Check sheet for the drawn part. Datum: minimum x, y, z corner. Units: mm. A direction names the side the tool comes from. Round coordinates to 2 decimals unless told otherwise and drop trailing zeros. Write each loop counter-clockwise with the first axis right and the second up, starting at its lowest first coordinate (ties: lowest second). Pieces come first, ordered by that corner, then holes. Notation, with made-up numbers: (-1.75, 18.25) - (42.25, 18.25) arc R28 ccw to (42.25, 42.25) - close; hole circle Ø4 at (-20.5, -22). An arc over 180 degrees is marked (long way). Answer as a JSON object with one key per item and string values. Group by question number.
Item 1: Sectioned sample at D-D on x = 12. Record the boundary of the cut face in (y, z) (1 decimal).
Item 2: Release check for a two-part mould opening along X. For the marked faces 1, 2 and 3 record: pulls with the +X half, pulls with the -X half, needs draft (parallel to the pull), parting line crosses it, or undercut.
Item 3: Sectioned sample at B-B on y = 4.75. Record the boundary of the cut face in (x, z).
Item 4: Set-up check for the marked faces 4, 5 and 6: record each of +Z, -Z, +X, -X, +Y, -Y from which the full face is reachable in a straight line by a thin tool's end or side.
Item 5: Sectioned sample at A-A on z = 5. Record the boundary of the cut face in (x, y).
Item 6: Thickness scan on line 1 (Y direction, x = 10, z = 12); line 2 (X direction, y = 9.5, z = 14) (1 decimal); line 3 (Z direction, x = 31, y = 17.75). Record the ranges inside material, lowest first.
Item 7: Gauge pin test, flat ends, axial feed: P1, Ø1.5, axis at y = 13, z = 6.5, coming from the -X side; P2, Ø11, axis at x = 29, y = 17.5, coming from the -Z side; P3, Ø1.5, axis at x = 38.5, z = 16, coming from the -Y side; P4, Ø0.6, axis at x = 21.5, z = 33.5, coming from the -Y side. Record the tip position at first contact, or that the pin passes through.
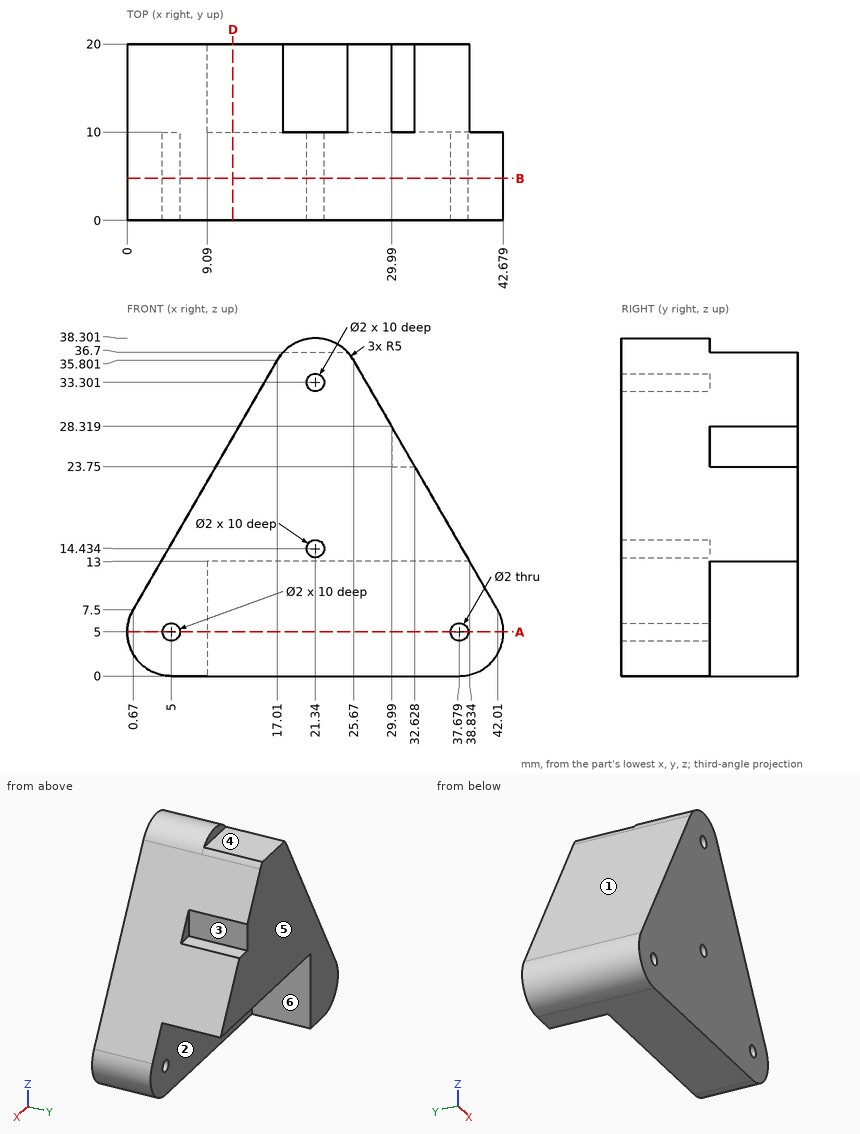
Completed:
{
 "1": {"outline": "(0, 0) - (10, 0) - (10, 13) - (20, 13) - (20, 27.1) - (0, 27.1) - close"},
 "2": {"face 1": "pulls with the -X half", "face 2": "needs draft", "face 3": "pulls with the +X half"},
 "3": {"outline": "(0.67, 7.5) arc R5 ccw to (5, 0) - (37.68, 0) arc R5 ccw to (42.01, 7.5) - (25.67, 35.8) arc R5 ccw to (17.01, 35.8) - close; hole circle Ø2 at (5, 5); hole circle Ø2 at (21.34, 14.43); hole circle Ø2 at (21.34, 33.3); hole circle Ø2 at (37.68, 5)"},
 "4": {"face 4": "+Z, +X, -X, +Y", "face 5": "+Z, -Z, +X, -X, +Y", "face 6": "-Z, +X, +Y"},
 "5": {"outline": "(0, 0) - (4, 0) - (4, 10) - (6, 10) - (6, 0) - (36.68, 0) - (36.68, 10) - (9.09, 10) - (9.09, 20) - (0, 20) - close; (38.68, 0) - (42.68, 0) - (42.68, 10) - (38.68, 10) - close"},
 "6": {"line 1": "0 to 10", "line 2": "4.4 to 20.4, 22.2 to 38.3", "line 3": "13 to 23.75"},
 "7": {"P1": "x = 0.06", "P2": "z = 13", "P3": "through", "P4": "y = 10"}
}
